```python
from build123d import *

# Parameters (mm, degrees)
F0_W     = 10
F0_H     = 7
F1_DEPTH = 24
F2_R     = 1.5
F3_DEPTH = 10


with BuildPart() as f1:
    # F0 (on Front) → F1 (new body)
    with BuildSketch(Plane.XZ):
        with BuildLine():
            Line((10, 0), (0, 0))
            ThreePointArc((0, 0), (5, -2.603278), (10, 0))
        make_face()
        with BuildLine():
            ThreePointArc((10, 7), (5, 9.603278), (0, 7))
            Line((0, 7), (10, 7))
        make_face()
        with Locations((5, 3.5)):
            Rectangle(F0_W, F0_H)
    extrude(amount=F1_DEPTH)

    # F2 (on face) → F3 (join)
    with BuildSketch(Plane.XZ.offset(24)):
        with Locations((5, 3.5)):
            Circle(F2_R)
    extrude(amount=F3_DEPTH)


solid = f1.part
```
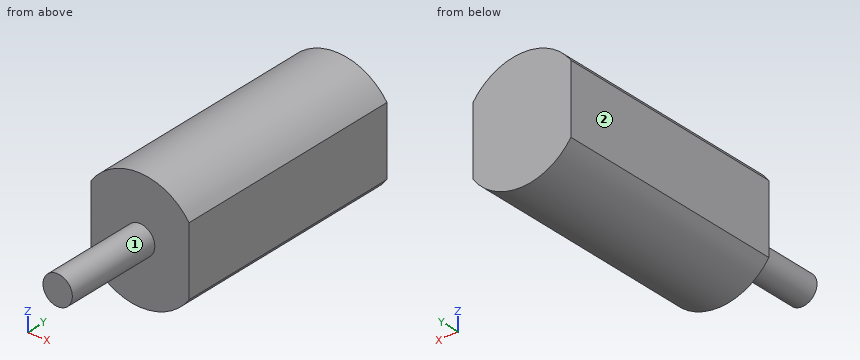
Verification items for the finished model (mm, model axes). Face numbers are marked on the shaded views. A direction names the side the tool comes from. Coordinates: 2 decimals unless noted, no trailing zeros. Order: outer loops, then holes, each group sorted by start corner. A loop starts at its lowest first (then second) coordinate and runs counter-clockwise, first axis right, second up. Notation, with made-up numbers: (-1.5, -8.5) -> (50.5, -8.5) arc R33 ccw to (50.5, 28.5) -> close; hole circle Ø5 at (31, -5.5). An arc over 180 degrees is marked (long way). Put each result on its own line as item: value. Start each with the question number.
1) Cross-section at C-C (y = -4). Enter the section's corners in (x, z).
2) Go/stop test with flat-tipped pins: pin 1 (1 mm diameter, centred on x = 7, y = -4, fed in from -Z); pin 2 (1.5 mm diameter, centred on x = 3.5, z = 7, fed in from -Y); pin 3 (1.5 mm diameter, centred on x = 7, z = -0.5, fed in from +Y); pin 4 (3 mm diameter, centred on x = 1.5, y = -9.5, fed in from +Z). Record where each tip stops, or that it passes through.
3) Tool access check on the marked faces 1 and 2. Record the directions out of +Z, -Z, +X, -X, +Y, -Y that give a thin tool (end or side, any length) a straight path to the whole face; none if there is none.
4) Cross-section at D-D (x = 1.5). Enter the section's corners in (y, z).
5) Material ranges on L1, parallel to Y at x = 9, z = 8; L2, parallel to Z at x = 2.25, y = -23.5; L3, parallel to X at y = -12.5, z = 8, recorded low to high.
6) Cross-section at B-B (x = 5). Enter the section's corners in (y, z), plus the area to 3 significant figures.
7) Cross-section at A-A (z = 3.5). Enter the section's corners in (x, y), plus the area to 3 significant figures.
Geometry check:
1. outline: (0, 0) arc R6.1 ccw to (10, 0) -> (10, 7) arc R6.1 ccw to (0, 7) -> close
2. pin 1: stops at z = -2.42
2. pin 2: stops at y = -24
2. pin 3: stops at y = 0
2. pin 4: stops at z = 9.27
3. face 1: -Y
3. face 2: +Z, -Z, -X, +Y, -Y
4. outline: (-24, -1.5) -> (0, -1.5) -> (0, 8.5) -> (-24, 8.5) -> close
5. L1: y = -24 to 0
5. L2: z = -1.95 to 8.95
5. L3: x = 0.88 to 9.12
6. outline: (-34, 2) -> (-24, 2) -> (-24, -2.6) -> (0, -2.6) -> (0, 9.6) -> (-24, 9.6) -> (-24, 5) -> (-34, 5) -> close
6. area: 323 mm^2
7. outline: (0, -24) -> (3.5, -24) -> (3.5, -34) -> (6.5, -34) -> (6.5, -24) -> (10, -24) -> (10, 0) -> (0, 0) -> close
7. area: 270 mm^2
